Work out the finished part from the listing and answer in its coordinate system (mm). Face numbers are marked on the shaded views. A direction names the side the tool comes from. Give positions to 0.01 mm unless a question says otherwise; leave off trailing zeros. Write each loop counter-clockwise with the first axis right and the second up, starting at its lowest first coordinate (ties: lowest second). Pieces come first, ordered by that corner, then holes. Notation, with made-up numbers: (53.25, -32.5) - (104.25, -32.5) arc R26 ccw to (104.25, -1.5) - close; hole circle Ø11 at (59.25, 63). An arc over 180 degrees is marked (long way). Write each question's results on one line, items separated by ' | '. Start each with the question number.
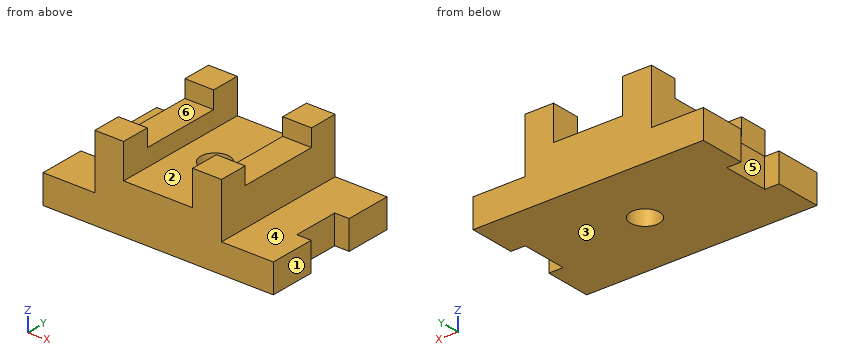
from build123d import *

# Parameters (mm, degrees)
F1_DEPTH  = 152.4
F2_W      = 15.875
F2_H      = 50.8
F3_DEPTH  = 31.751
F4_W      = 15.875
F4_H      = 50.8
F5_DEPTH  = 31.751
F6_W      = 76.2
F6_H      = 152.4
F7_DEPTH  = 19.05
F9_W      = 31.75
F9_H      = 88.9
F10_DEPTH = 19.05
F8_W      = 31.75
F8_H      = 88.9
F11_DEPTH = 19.05
F12_R     = 15.875
F13_DEPTH = 53.976


with BuildPart() as f1:
    # F0 (on Front) → F1 (new body)
    with BuildSketch(Plane.XZ):
        Polygon((-127, 0), (0, 0), (0, 31.75), (-57.15, 31.75), (-57.15, 92.075), (-88.9, 92.075), (-88.9, 73.025), (-165.1, 73.025), (-165.1, 92.075), (-196.85, 92.075), (-196.85, 31.75), (-254, 31.75), (-254, 0), align=None)
    extrude(amount=F1_DEPTH)

    # F2 (on face) → F3 (cut, through all)
    with BuildSketch(Plane.XY.offset(31.75)):
        with Locations((-7.9375, -76.2)):
            Rectangle(F2_W, F2_H)
    extrude(amount=-F3_DEPTH, mode=Mode.SUBTRACT)

    # F4 (on face) → F5 (cut, through all)
    with BuildSketch(Plane.XY.offset(31.75)):
        with Locations((-246.0625, -76.2)):
            Rectangle(F4_W, F4_H)
    extrude(amount=-F5_DEPTH, mode=Mode.SUBTRACT)

    # F6 (on face) → F7 (cut)
    with BuildSketch(Plane.XY.offset(73.025)):
        with Locations((-127, -76.2)):
            Rectangle(F6_W, F6_H)
    extrude(amount=-F7_DEPTH, mode=Mode.SUBTRACT)

    # F9 (on face) → F10 (cut)
    with BuildSketch(Plane.XY.offset(92.075)):
        with Locations((-73.025, -76.2)):
            Rectangle(F9_W, F9_H)
    extrude(amount=-F10_DEPTH, mode=Mode.SUBTRACT)

    # F8 (on face) → F11 (cut)
    with BuildSketch(Plane.XY.offset(92.075)):
        with Locations((-180.975, -76.2)):
            Rectangle(F8_W, F8_H)
    extrude(amount=-F11_DEPTH, mode=Mode.SUBTRACT)

    # F12 (on face) → F13 (cut, through all)
    with BuildSketch(Plane.XY.offset(53.975)):
        with Locations((-127, -76.2)):
            Circle(F12_R)
    extrude(amount=-F13_DEPTH, mode=Mode.SUBTRACT)


solid = f1.part
Q1. A cutting plane is placed at A-A, the plane x = -127. Write down the section's boundary in (y, z) (3 decimals), and give its area (3 significant figures).
Q2. A cutting plane is placed at D-D, the plane y = -25.5. Write down the section's boundary in (x, z) (3 decimals).
Q3. Consider L1, parallel to Y at x = -127, z = 27 (3 decimals); L2, parallel to X at y = -76, z = 18 (3 decimals); L3, parallel to Y at x = -170.5, z = 88.5. Determine where each line is inside the solid, lowest interval first.
Q4. Given pin 1 (10 mm diameter, centred on y = -94, z = 26, fed in from -X) (3 decimals); pin 2 (16 mm diameter, centred on y = -67, z = 15.5, fed in from +X) (3 decimals); pin 3 (18 mm diameter, centred on y = -78, z = 55.5, fed in from +X), each flat-ended and moving along its own axis, determine where each tip first touches the part or whether it passes through.
Q5. A tool of negligible diameter and unlimited length cuts with its end or side. For the marked faces 4, 5 and 6, from which of +Z, -Z, +X, -X, +Y, -Y can it reach the whole face along a straight path? Write none if from no direction.
Q6. The mould has two halves that part along X. Classify the marked faces 1, 2 and 3: pulls with the +X half, pulls with the -X half, needs draft (parallel to the pull), parting line crosses it, or undercut.
Q7. A cutting plane is placed at B-B, the plane z = 60. Write down the section's boundary in (x, y).
Q8. A cutting plane is placed at C-C, the plane y = -76.2. Write down the section's boundary in (x, z) (3 decimals), and give its area (3 significant figures).
Result:
1) outline: (-152.4, 0) - (-92.075, 0) - (-92.075, 53.975) - (-152.4, 53.975) - close; (-60.325, 0) - (0, 0) - (0, 53.975) - (-60.325, 53.975) - close | area: 6,510 mm2
2) outline: (-254, 0) - (0, 0) - (0, 31.75) - (-57.15, 31.75) - (-57.15, 92.075) - (-88.9, 92.075) - (-88.9, 53.975) - (-165.1, 53.975) - (-165.1, 92.075) - (-196.85, 92.075) - (-196.85, 31.75) - (-254, 31.75) - close
3) L1: y = -152.4 to -92.075, -60.325 to 0 | L2: x = -238.125 to -142.874, -111.126 to -15.875 | L3: y = -152.4 to -120.65, -31.75 to 0
4) pin 1: stops at x = -238.125 | pin 2: stops at x = -15.875 | pin 3: stops at x = -57.15
5) face 4: +Z, +X, +Y, -Y | face 5: +Z, -Z, -X | face 6: +Z, +X, -X
6) face 1: pulls with the +X half | face 2: undercut | face 3: needs draft
7) outline: (-196.85, -152.4) - (-165.1, -152.4) - (-165.1, 0) - (-196.85, 0) - close; (-88.9, -152.4) - (-57.15, -152.4) - (-57.15, 0) - (-88.9, 0) - close
8) outline: (-238.125, 0) - (-142.875, 0) - (-142.875, 53.975) - (-165.1, 53.975) - (-165.1, 73.025) - (-196.85, 73.025) - (-196.85, 31.75) - (-238.125, 31.75) - close; (-111.125, 0) - (-15.875, 0) - (-15.875, 31.75) - (-57.15, 31.75) - (-57.15, 73.025) - (-88.9, 73.025) - (-88.9, 53.975) - (-111.125, 53.975) - close | area: 9,660 mm2
